Build history of the part. All positions in model axes, mm. Round coordinates to 2 decimals unless told otherwise and drop trailing zeros. Order: outer loops, then holes, each group sorted by start corner. A loop starts at its lowest first (then second) coordinate and runs counter-clockwise, first axis right, second up. Notation, with made-up numbers: M -39.75,-3.75 L -11.75,-3.75 A23 cw -11.75,29.25 Z; hole C -16.75,-38.5 d2. An arc over 180 degrees is marked long. One line per item, written item: value. Start each with the question number.
Item 1: Band-saw the part on A-A, the plane x = -485. Write the cut outline in (y, z), then the cut area to 3 significant figures.
Item 2: Probe L1, parallel to Z at x = -523, y = -0.7; L2, parallel to Y at x = -182.5, z = -12.5. List the from-to ranges inside material, lowest first.
Item 3: Pin check, flat tips, straight feed: pin 1 (1.5 mm diameter, centred on x = -489.5, z = 10.5, fed in from +Y); pin 2 (1.5 mm diameter, centred on x = 165, z = 18.5, fed in from +Y). Stop position of each tip, or through.
Item 4: Band-saw the part on B-B, the plane y = -0.7. Write the cut outline in (x, z).
```python
from build123d import *

# Parameters (mm, degrees)
F0_W     = 1380
F0_H     = 40
F1_DEPTH = 3
F2_W     = 1380
F2_H     = 5
F2_H_2   = 10
F3_DEPTH = 1.5
F4_R     = 2


with BuildPart() as f1:
    # F0 (on Front) → F1 (new body)
    with BuildSketch(Plane.XZ):
        Rectangle(F0_W, F0_H)
    extrude(amount=F1_DEPTH)

    # F2 (on face) → F3 (cut)
    with BuildSketch(Plane(origin=(0, 0, 0), x_dir=(-1, 0, 0), z_dir=(0, 1, 0))):
        with Locations((0, 17.5)):
            Rectangle(F2_W, F2_H)
        with Locations((0, -15)):
            Rectangle(F2_W, F2_H_2)
    extrude(amount=-F3_DEPTH, mode=Mode.SUBTRACT)

    # F4
    f4_edges = [f1.edges().sort_by_distance(p)[0] for p in [
        (690, -2.25, 20),
        (690, -2.25, -20),
        (-690, -2.25, 20),
        (-690, -2.25, -20),
    ]]
    fillet(f4_edges, radius=F4_R)


solid = f1.part
```
Output:
1. outline: M -3,-20 L -1.5,-20 L -1.5,-10 L 0,-10 L 0,15 L -1.5,15 L -1.5,20 L -3,20 Z
1. area: 97.5 mm²
2. L1: z = -10 to 15
2. L2: y = -3 to -1.5
3. pin 1: stops at y = 0
3. pin 2: stops at y = -1.5
4. outline: M -690,-10 L 690,-10 L 690,15 L -690,15 Z
